For this review, take the finished solid that the model builds, in its own axes (mm). A direction names the side the tool comes from. Round coordinates to 2 decimals unless told otherwise and drop trailing zeros. Write each loop counter-clockwise with the first axis right and the second up, starting at its lowest first coordinate (ties: lowest second). Pieces come first, ordered by that corner, then holes.
from build123d import *

# Parameters (mm, degrees)
SKETCH2_W           = 20
SKETCH2_H           = 20
BOSS_EXTRUDE1_DEPTH = 20
SKETCH3_R           = 2.25
CUT_EXTRUDE1_DEPTH  = 20
CUT_EXTRUDE2_DEPTH  = 3.3
FILLET1_R           = 3


with BuildPart() as part:
    # Sketch1 → Revolve1 (revolve)
    with BuildSketch(Plane(origin=(0, 0, 0), x_dir=(1, 0, 0), z_dir=(0, 1, 0))):
        with BuildLine():
            Line((0, 15), (0, -15))
            ThreePointArc((0, -15), (-15, 0), (0, 15))
        make_face()
    revolve(axis=Axis((0, 0, -15), (0, 0, 1)))

    # Sketch2 → Boss-Extrude1 (add)
    with BuildSketch(Plane.XY):
        Rectangle(SKETCH2_W, SKETCH2_H)
    extrude(amount=BOSS_EXTRUDE1_DEPTH)

    # Sketch3 → Cut-Extrude1 (cut)
    with BuildSketch(Plane.XY.offset(20)):
        Circle(SKETCH3_R)
    extrude(amount=-CUT_EXTRUDE1_DEPTH, mode=Mode.SUBTRACT)

    # Sketch4 → Cut-Extrude2 (cut)
    with BuildSketch(Plane.XY.offset(15)):
        Polygon((2.165063509, 3.75), (10, 3.75), (10, -3.75), (2.165063509, -3.75), (-2.165063509, -3.75), (-4.330127019, 0), (-2.165063509, 3.75), align=None)
    extrude(amount=-CUT_EXTRUDE2_DEPTH, mode=Mode.SUBTRACT)

    # Fillet1
    fillet1_edges = [part.edges().sort_by_distance(p)[0] for p in [
        (10, -10, 12.5),
        (10, 10, 12.5),
        (-10, 10, 12.5),
        (-10, -10, 12.5),
    ]]
    fillet(fillet1_edges, radius=FILLET1_R)


solid = part.part
(1) For pin 1 Ø8 at (x, y) = (0.5, -2) entering from -Z; pin 2 Ø3 at (x, z) = (-8, 7) entering from -Y; pin 3 Ø12.5 at (x, z) = (0.5, 16) entering from +Y; pin 4 Ø3.5 at (y, z) = (3, 17) entering from +X, all flat-tipped, find the tip position at first contact; note any pin that passes through.
Geometry check:
pin 1: stops at z = -15
pin 2: stops at y = -11.9
pin 3: stops at y = 11.39
pin 4: stops at x = 10
(2) We need section B-B, the plane x = 0. Give the boundary of the cut face in (y, z), and give its area (3 significant figures).
Geometry check:
outline: (-10, 11.18) arc R15 ccw (long way) to (10, 11.18) - (10, 20) - (2.25, 20) - (2.25, 15) - (3.75, 15) - (3.75, 11.7) - (2.25, 11.7) - (2.25, 0) - (-2.25, 0) - (-2.25, 11.7) - (-3.75, 11.7) - (-3.75, 15) - (-2.25, 15) - (-2.25, 20) - (-10, 20) - close
area: 731 mm2
(3) We need section C-C, the plane z = 4.5. Give the boundary of the cut face in (x, y), and give its area (3 significant figures).
Geometry check:
outline: circle Ø28.62 at (0, 0); hole circle Ø4.5 at (0, 0)
area: 627 mm2
(4) We need section D-D, the plane y = 9.5. Give the boundary of the cut face in (x, z), and give its area (3 significant figures).
Geometry check:
outline: (-8.66, 7.73) arc R11.61 ccw (long way) to (8.66, 7.73) - (8.66, 20) - (-8.66, 20) - close
area: 589 mm2
(5) We need section A-A, the plane x = 4.5. Give the boundary of the cut face in (y, z).
Geometry check:
outline: (-10, 10.23) arc R14.31 ccw (long way) to (10, 10.23) - (10, 20) - (-10, 20) - close; hole (-3.75, 11.7) - (3.75, 11.7) - (3.75, 15) - (-3.75, 15) - close
(6) For line 1 along Y through (x, z) = (0, 16.4); line 2 along Z through (x, y) = (5.75, 3); line 3 along Z through (x, y) = (9.5, -3), list the stretches that pass through material, from the lowest coordinate up.
Geometry check:
line 1: y = -10 to -2.25, 2.25 to 10
line 2: z = -13.53 to 11.7, 15 to 20
line 3: z = -11.21 to 11.7, 15 to 20
(7) Mouldability with a two-part tool opening along X and no side actions: class faces 1 (the face through (-9.14, -9.1, 13.91)), 2 (the face through (-0.29, 2.23, 17.54)), 3 (the face through (-3.232, -1.901, 13.373)) as pulls with the +X half, pulls with the -X half, needs draft (parallel to the pull), parting line crosses it, or undercut.
Geometry check:
face 1: pulls with the -X half
face 2: undercut
face 3: pulls with the +X half
(8) For faces 4 (the face through (-0.29, 2.23, 5.93)), 5 (the face through (5, 0, 15)), 6 (the face through (9.1, -9.14, 13.91)), 7 (the face through (-9.14, 9.1, 13.91)), list the 3-axis set-ups (+Z, -Z, +X, -X, +Y, -Y) from which the entire face can be reached by the end or side of a thin tool; tool diameter is ignored.
Geometry check:
face 4: +Z
face 5: +X
face 6: +Z, +X, -Y
face 7: +Z, -X, +Y
